Verification items for the finished model (mm, model axes). Face numbers are marked on the shaded views. Give positions to 0.01 mm unless a question says otherwise; leave off trailing zeros. Write each loop counter-clockwise with the first axis right and the second up, starting at its lowest first coordinate (ties: lowest second). Pieces come first, ordered by that corner, then holes.
from build123d import *

# Parameters (mm, degrees)
F0_R     = 3.55
F1_DEPTH = 25
F2_SIZE2 = 19.0811366877
F2_SIZE  = 1
F3_R     = 4.5061105162
F4_DEPTH = 15
F5_R     = 1.5
F6_DEPTH = 25


with BuildPart() as f1:
    # F0 (on Front) → F1 (new body)
    with BuildSketch(Plane.XZ):
        with Locations((-36.0824763775, 37.0747447014)):
            Circle(F0_R)
    extrude(amount=F1_DEPTH)

    # F2
    f2_edges = [f1.edges().sort_by_distance(p)[0] for p in [
        (-39.632476, -25, 37.074745),
    ]]
    f2_side = f1.faces().sort_by_distance((-36.082476, -25, 37.074745))[0]
    chamfer(f2_edges, length=F2_SIZE, length2=F2_SIZE2, reference=f2_side)

    # F3 (on face) → F4 (cut)
    with BuildSketch(Plane.XZ.offset(25)):
        with Locations((-36.0824763775, 37.0747447014)):
            Circle(F3_R)
    extrude(amount=-F4_DEPTH, mode=Mode.SUBTRACT)

    # F5 (on face) → F6 (cut)
    with BuildSketch(Plane.XZ.offset(10)):
        with Locations((-36.0824763775, 37.0747447014)):
            Circle(F5_R)
    extrude(amount=-F6_DEPTH, mode=Mode.SUBTRACT)


solid = f1.part
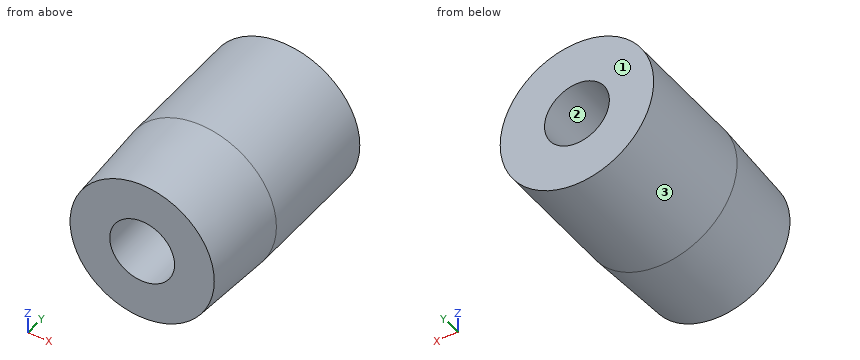
Item 1: Scan lines: line 1 along Z through (x, y) = (-36, -1.5); line 2 along X through (y, z) = (-5.75, 37.5); line 3 along X through (y, z) = (-6.25, 38.25). Record each from-to range of solid material in increasing order.
Answer key:
line 1: z = 33.53 to 35.58, 38.57 to 40.62
line 2: x = -39.61 to -37.52, -34.64 to -32.56
line 3: x = -39.41 to -37.01, -35.15 to -32.75
Item 2: Sectioned sample at A-A on y = -7.25. Record the cut outline in (x, z), then the cut area to 3 significant figures.
Answer key:
outline: circle Ø6.96 at (-36.08, 37.07); hole circle Ø3 at (-36.08, 37.07)
area: 31.0 mm2
Item 3: Sectioned sample at B-B on y = -8.75. Record the cut outline in (x, z), then the cut area to 3 significant figures.
Answer key:
outline: circle Ø6.8 at (-36.08, 37.07); hole circle Ø3 at (-36.08, 37.07)
area: 29.3 mm2
Item 4: Release check for a two-part mould opening along X. For the marked faces 1, 2 and 3 record: released by +X, released by -X, zero draft, split by the parting line, or undercut.
Answer key:
face 1: zero draft
face 2: undercut
face 3: split by the parting line
Item 5: Depth check by flat-ended pin: pin 1 (3 mm diameter, centred on y = -6.5, z = 39, fed in from -X); pin 2 (1.8 mm diameter, centred on x = -36.08, z = 37.07, fed in from -Y); pin 3 (1 mm diameter, centred on x = -36, y = -8, fed in from +Z). Enter the tip coordinate at first touch or a pass-through.
Answer key:
pin 1: stops at x = -39.59
pin 2: passes through
pin 3: stops at z = 40.54
